Source: CAD feature listing. Evaluate the final solid. Frame: model axes, mm. A direction names the side the tool comes from. Round coordinates to 2 decimals unless told otherwise and drop trailing zeros. Order: outer loops, then holes, each group sorted by start corner. A loop starts at its lowest first (then second) coordinate and runs counter-clockwise, first axis right, second up.
```python
from build123d import *

# Parameters (mm, degrees)
SKETCH1_R           = 1.6000000000000016
BOSS_EXTRUDE1_DEPTH = 15.239999999999998
SKETCH2_R           = 4.8260000000000005
CUT_EXTRUDE1_DEPTH  = 4.0005
FILLET2_R           = 2.54
FILLET3_R           = 2.54


with BuildPart() as part:
    # Sketch1 → Boss-Extrude1 (new body)
    with BuildSketch(Plane(origin=(0, 0, 0), x_dir=(1, 0, 0), z_dir=(0, 1, 0))):
        with BuildLine():
            Line((-19.782278512640783, -6.1e-16), (-13.782278512640788, 0))
            Line((-13.782278512640788, 0), (-1.6509999999999998, 0))
            ThreePointArc((-1.651, -4.2e-16), (-3.8e-16, 1.6509999999999998), (1.6509999999999996, 0))
            Line((1.6509999999999998, 0), (15.624999999999998, -1.4e-16))
            ThreePointArc((15.625, -1.4e-16), (22.584560100693558, -3.665380266766327), (21.670000000000005, 4.147050156436503))
            Line((21.67, 4.147050156436504), (21.67, 8.211050156436503))
            Line((21.67, 8.211050156436503), (11.769870701434405, 8.211050156436503))
            ThreePointArc((11.769870701434405, 8.211050156436505), (6.637560553583663, 12.723756949011177), (2.2e-16, 14.351))
            ThreePointArc((8.9e-16, 14.350999999999999), (-8.618213300911037, 11.475086078108522), (-13.782278512640787, 4.000000000000001))
            Line((-13.782278512640788, 4), (-16.782278512640787, 4))
            Line((-16.782278512640787, 4), (-16.782278512640787, 6))
            Line((-16.782278512640787, 6), (-19.782278512640783, 4))
            Line((-19.782278512640783, 4), (-19.782278512640783, -6.1e-16))
        make_face()
        with Locations(Location((20.07, 8e-16, 0), (0, 0, 90))):
            Circle(SKETCH1_R, mode=Mode.SUBTRACT)
    extrude(amount=BOSS_EXTRUDE1_DEPTH)

    # Sketch2 → Cut-Extrude1 (cut, symmetric)
    with BuildSketch(Plane(origin=(0, 7.619999999999999, 0), x_dir=(1, 0, 0), z_dir=(0, 1, 0))):
        with Locations((20.07, 8e-16)):
            Circle(SKETCH2_R)
    extrude(amount=CUT_EXTRUDE1_DEPTH, both=True, mode=Mode.SUBTRACT)

    # Fillet2
    fillet2_edges = [part.edges().sort_by_distance(p)[0] for p in [
        (-3.8e-16, 15.239999999999998, -1.6509999999999998),
    ]]
    fillet(fillet2_edges, radius=FILLET2_R)

    # Fillet3
    fillet3_edges = [part.edges().sort_by_distance(p)[0] for p in [
        (21.67, 1.8097499999999997, -4.147050156436503),
    ]]
    fillet(fillet3_edges, radius=FILLET3_R)


solid = part.part
```
1. Section C-C on x = 0. Return loops of the section in (y, z).
2. Section A-A on x = 20.07. Return loops of the section in (y, z) (1 decimal), plus the area to 3 significant figures.
3. Pull-direction query (X, two-part tool) for faces 1 (the face through (-15, 8, -4)), 2 (the face through (21.67, 8, -7)), 3 (the face through (2, 15.24, -5)); classes: released by +X, released by -X, zero draft, split by the parting line, or undercut.
4. Line query: line 1 along Z through (x, y) = (0, 6); line 2 along Z through (x, y) = (20.07, 14.25) (3 decimals); line 3 along X through (y, z) = (5.5, -5.5). Output: solid intervals per line, ascending.
5. Section D-D on z = -12.25. Return loops of the section in (x, y).
6. First-contact query: pin 1 (3 mm diameter, centred on x = 10.5, y = 12, fed in from -Z); pin 2 (3 mm diameter, centred on y = 5, z = -7, fed in from +X); pin 3 (7 mm diameter, centred on x = 9.5, y = 8, fed in from +Z); pin 4 (1.9 mm diameter, centred on x = 20.07, z = 0, fed in from +Y). Flat tips, straight axial feed; report the tip coordinate or a pass-through.
7. Section B-B on y = 9.75. Return loops of the section in (x, z), plus the area to 3 significant figures.
8. Access query for faces 4 (the face through (-11, 8, 0)), 5 (the face through (17.466, 7.676, -4.063)), 6 (the face through (-16.782, 8, -5)). Directions: +Z, -Z, +X, -X, +Y, -Y. A direction counts if a zero-diameter tool reaches every point of the face in a straight line with its end or side. Return the directions, or none.
Result:
1. outline: (0, -14.35) - (15.24, -14.35) - (15.24, -4.19) arc R2.54 ccw to (12.7, -1.65) - (0, -1.65) - close
2. outline: (0, -8.2) - (15.2, -8.2) - (15.2, -1.6) - (11.6, -1.6) - (11.6, -4.8) - (3.6, -4.8) - (3.6, -1.6) - (0, -1.6) - close; (0, 1.6) - (3.6, 1.6) - (3.6, 4.4) - (0, 4.4) - close; (11.6, 1.6) - (15.2, 1.6) - (15.2, 4.4) - (11.6, 4.4) - close
2. area: 95.5 mm2
3. face 1: undercut
3. face 2: released by +X
3. face 3: zero draft
4. line 1: z = -14.35 to -1.65
4. line 2: z = -8.211 to -1.6, 1.6 to 4.445
4. line 3: x = -17.53 to -16.78, -13.26 to 21.67
5. outline: (-7.48, 0) - (7.48, 0) - (7.48, 15.24) - (-7.48, 15.24) - close
6. pin 1: stops at z = -11.18
6. pin 2: stops at x = 21.67
6. pin 3: stops at z = 0
6. pin 4: passes through
7. outline: (-19.78, -4) - (-16.78, -6) - (-16.78, -4) - (-13.78, -4) arc R14.35 ccw to (11.77, -8.21) - (21.67, -8.21) - (21.67, -5.63) arc R2.54 cw to (21.96, -4.44) arc R4.83 cw to (15.24, 0) - (1.65, 0) arc R1.65 cw to (-1.65, 0) - (-19.78, 0) - close
7. area: 386 mm2
8. face 4: +Z, -X, +Y, -Y
8. face 5: +Z
8. face 6: -Z, +Y, -Y
